Geometry: final body of the model. Coordinates: model frame, mm. A direction names the side the tool comes from. Give positions to 0.01 mm unless a question says otherwise; leave off trailing zeros. Write each loop counter-clockwise with the first axis right and the second up, starting at its lowest first coordinate (ties: lowest second). Pieces come first, ordered by that corner, then holes. Notation, with made-up numbers: (36, 49.5) - (85, 49.5) arc R6 cw to (85, 60.5) - close; hole circle Ø1 at (8.25, 31.5). An arc over 180 degrees is marked (long way). Return JSON: item names as keys, results as strings.
Autodesk Inventor part; units mm, degrees
ref_plane "YZ Plane" through (0, 0, 0) normal (1, 0, 0) x (0, 1, 0)
ref_plane "XZ Plane" through (0, 0, 0) normal (0, 1, 0) x (-1, 0, 0)
ref_plane "XY Plane" through (0, 0, 0) normal (0, 0, 1) x (1, 0, 0)
sketch "Sketch3" plane through (0, 0, 0) normal (0, 0, 1) x (1, 0, 0)
  circle A0 centre (0, 0) radius 12.5
  dimension "d9" = 25
extrude "Extrusion3" add sketch "Sketch3" against normal blind 4
chamfer "Chamfer2" distance 0.5 angle 45 2 edges at (-12.5, 0, 0) (-12.5, 0, -4)
sketch "Sketch4" plane through (0, 0, -4) normal (0, 0, -1) x (-1, 0, 0)
  circle A0 centre (0, 0) radius 15
  dimension "d15" = 30
extrude "Extrusion4" add sketch "Sketch4" along normal blind 5
properties part number "Mirror"
Q1. Material intervals for probe 1 along Z at (x, y) = (0.25, 13); probe 2 along Y at (x, z) = (1.25, -2.25); probe 3 along Y at (x, z) = (-9.25, -1.5), sorted ascending. Write a range as [from, to].
Answer key:
{"probe 1": "z = [-9, -4]", "probe 2": "y = [-12.44, 12.44]", "probe 3": "y = [-8.41, 8.41]"}
Q2. Pin query (flat end, axial travel): P1, Ø6, axis at x = -11.5, y = 11, coming from the +Z side; P2, Ø4, axis at y = -8, z = -2.5, coming from the -X side; P3, Ø2, axis at y = -5, z = -4.5, coming from the -X side. Return the tip coordinate at first contact, or that it passes through.
Answer key:
{"P1": "stops at z = -4", "P2": "stops at x = -13.43", "P3": "stops at x = -14.46"}
Q3. Section query C-C, the plane z = -5.5. Return the cut outline in (x, y).
Answer key:
{"outline": "circle Ø30 at (0, 0)"}
Q4. Section query D-D, the plane z = -3. Return the cut outline in (x, y).
Answer key:
{"outline": "circle Ø25 at (0, 0)"}
Q5. Section query A-A, the plane x = 0. Return the cut outline in (y, z), plus the area to 4 significant figures.
Answer key:
{"outline": "(-15, -9) - (15, -9) - (15, -4) - (12, -4) - (12.5, -3.5) - (12.5, -0.5) - (12, 0) - (-12, 0) - (-12.5, -0.5) - (-12.5, -3.5) - (-12, -4) - (-15, -4) - close", "area": "249.5 mm^2"}
Q6. Set-up query: faces 1 (the flat face through (0.1, 12.3, -4)), 2 (the flat face through (0, 0, -9)), 3 (the cylindrical face through (11.923, 3.755, -1.979)). Return all of +Z, -Z, +X, -X, +Y, -Y with unobstructed straight access to the full face (end or side cutting, diameter ignored); none if empty.
Answer key:
{"face 1": "none", "face 2": "-Z, +X, -X, +Y, -Y", "face 3": "+Z"}
